Geometry check sheet. Reference: the model listing, model coordinates, mm. Face numbers are marked on the shaded views. A direction names the side the tool comes from. Round coordinates to 2 decimals unless told otherwise and drop trailing zeros. Write each loop counter-clockwise with the first axis right and the second up, starting at its lowest first coordinate (ties: lowest second). Pieces come first, ordered by that corner, then holes. Notation, with made-up numbers: (41, 2.5) -> (51, 2.5) arc R20 ccw to (51, 11.5) -> close; hole circle Ø2 at (-20, 65). An arc over 180 degrees is marked (long way). Use a Markdown table: item, result.
```python
from build123d import *

# Parameters (mm, degrees)
SKETCH_1_R      = 1.25
EXTRUDE_1_DEPTH = 12
FILLET_1_R      = 1


with BuildPart() as part:
    # 草图1 → 凸台-拉伸1 (new body)
    with BuildSketch(Plane.XY):
        Polygon((0, 0), (21, 0), (21, -10), (31, -10), (31, -40), (0, -40), (0, -20), (7, -17.5), (14, -17.5), (14, -12.5), (7, -12.5), (0, -10), align=None)
        with Locations((7, -6)):
            Circle(SKETCH_1_R, mode=Mode.SUBTRACT)
        with Locations((23, -15)):
            Circle(SKETCH_1_R, mode=Mode.SUBTRACT)
        with Locations((7, -24.5)):
            Circle(SKETCH_1_R, mode=Mode.SUBTRACT)
    extrude(amount=EXTRUDE_1_DEPTH)

    # 圆角1
    fillet_1_edges = [part.edges().sort_by_distance(p)[0] for p in [
        (10.5, 0, 0),
        (26, -10, 0),
        (31, -25, 0),
        (15.5, -40, 0),
        (0, -30, 0),
        (0, -5, 0),
        (0, 0, 6),
        (21, 0, 6),
        (31, -10, 6),
        (31, -40, 6),
        (0, -40, 6),
        (14, -17.5, 6),
        (14, -12.5, 6),
        (0, -30, 12),
        (15.5, -40, 12),
        (31, -25, 12),
        (26, -10, 12),
        (10.5, 0, 12),
        (0, -5, 12),
    ]]
    fillet(fillet_1_edges, radius=FILLET_1_R)


solid = part.part
```
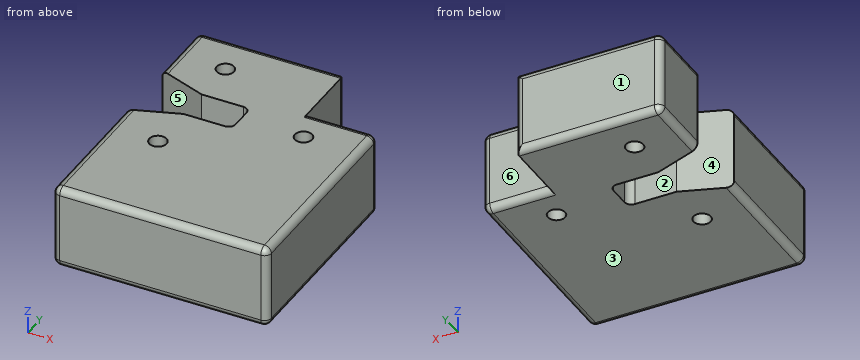
(1) Section check B-B on x = 23. Record the cut outline in (y, z).
A:
| item | result |
|---|---|
| outline | (-40, 1) arc R1 ccw to (-39, 0) -> (-16.25, 0) -> (-16.25, 12) -> (-39, 12) arc R1 ccw to (-40, 11) -> close; (-13.75, 0) -> (-11, 0) arc R1 ccw to (-10, 1) -> (-10, 11) arc R1 ccw to (-11, 12) -> (-13.75, 12) -> close |
(2) Section check A-A on y = -15. Record the cut outline in (x, z).
A:
| item | result |
|---|---|
| outline | (14, 0) -> (21.75, 0) -> (21.75, 12) -> (14, 12) -> close; (24.25, 0) -> (30, 0) arc R1 ccw to (31, 1) -> (31, 11) arc R1 ccw to (30, 12) -> (24.25, 12) -> close |
(3) Gauge pin test, flat end, axial feed: pin 1 Ø3.5 at (y, z) = (-15.5, 8.5) entering from -X. Record the tip position at first contact, or that the pin passes through.
A:
| item | result |
|---|---|
| pin 1 | stops at x = 13.66 |
(4) Thickness scan on line 1 (Y direction, x = 7, z = 3.5); line 2 (Y direction, x = 11, z = 10.75); line 3 (Y direction, x = 23, z = 8.5). Record the ranges inside material, lowest first.
A:
| item | result |
|---|---|
| line 1 | y = -40 to -25.75, -23.25 to -17.5, -12.5 to -7.25, -4.75 to 0 |
| line 2 | y = -40 to -17.5, -12.5 to 0 |
| line 3 | y = -40 to -16.25, -13.75 to -10 |
(5) Access from +Z, -Z, +X, -X, +Y, -Y to the whole of each face (thin tool, end or side, straight path). Record for the marked faces 1 and 2.
A:
| item | result |
|---|---|
| face 1 | +Z, -Z, +X, -X, +Y |
| face 2 | +Z, -Z, -X |
(6) Section check C-C on x = 27. Record the cut outline in (y, z).
A:
| item | result |
|---|---|
| outline | (-40, 1) arc R1 ccw to (-39, 0) -> (-11, 0) arc R1 ccw to (-10, 1) -> (-10, 11) arc R1 ccw to (-11, 12) -> (-39, 12) arc R1 ccw to (-40, 11) -> close |
(7) Release check for a two-part mould opening along Y. For the marked faces 3, 4, 5 and 6 record: +Y half, -Y half, draft (parallel to the pull), parting line (faces both ways), or undercut.
A:
| item | result |
|---|---|
| face 3 | draft |
| face 4 | undercut |
| face 5 | undercut |
| face 6 | +Y half |
(8) Section check D-D on z = 5.25. Record the cut outline in (x, y), plus the area to 3 significant figures.
A:
| item | result |
|---|---|
| outline | (0, -39) arc R1 ccw to (1, -40) -> (30, -40) arc R1 ccw to (31, -39) -> (31, -11) arc R1 ccw to (30, -10) -> (21, -10) -> (21, -1) arc R1 ccw to (20, 0) -> (1, 0) arc R1 ccw to (0, -1) -> (0, -10) -> (7, -12.5) -> (13, -12.5) arc R1 cw to (14, -13.5) -> (14, -16.5) arc R1 cw to (13, -17.5) -> (7, -17.5) -> (0, -20) -> close; hole circle Ø2.5 at (7, -24.5); hole circle Ø2.5 at (7, -6); hole circle Ø2.5 at (23, -15) |
| area | 1,040 mm2 |
